from build123d import *

# Parameters (mm, degrees)
F0_W     = 127
F0_H     = 127
F1_DEPTH = 127
F2_W     = 38.1
F2_H     = 38.1
F3_DEPTH = 25.4
F4_W     = 88.9
F4_H     = 25.4
F5_DEPTH = 50.8
F6_W     = 25.4
F6_H     = 25.4
F7_DEPTH = 63.5
F8_W     = 12.7
F8_H     = 12.7
F9_DEPTH = 10.16


with BuildPart() as f1:
    # F0 (on Front) → F1 (new body)
    with BuildSketch(Plane.XZ):
        Rectangle(F0_W, F0_H)
    extrude(amount=F1_DEPTH)

    # F2 (on face) → F3 (join)
    with BuildSketch(Plane.XZ.offset(127)):
        with Locations((-44.45, -44.45)):
            Rectangle(F2_W, F2_H)
        with Locations((44.45, -44.45)):
            Rectangle(F2_W, F2_H)
    extrude(amount=F3_DEPTH)

    # F4 (on face) → F5 (join)
    with BuildSketch(Plane.XZ.offset(127)):
        with Locations((0, 76.2)):
            Rectangle(F4_W, F4_H)
        with Locations((0, 50.8)):
            Rectangle(F4_W, F4_H)
    extrude(amount=F5_DEPTH)

    # F6 (on face) → F7 (join)
    with BuildSketch(Plane.XY.offset(88.9)):
        with Locations((-31.75, -139.7)):
            Rectangle(F6_W, F6_H)
        with Locations((31.75, -139.7)):
            Rectangle(F6_W, F6_H)
    extrude(amount=F7_DEPTH)

    # F8 (on face) → F9 (join)
    with BuildSketch(Plane.XZ.offset(177.8)):
        with Locations((0, 62.430865)):
            Rectangle(F8_W, F8_H)
    extrude(amount=F9_DEPTH)


solid = f1.part
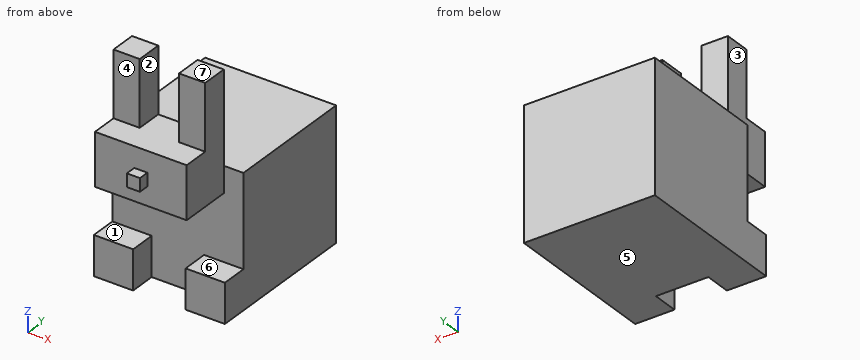
Read the model definition and answer for the solid it produces. Units are mm, in the model's axes. Face numbers are marked on the shaded views. A direction names the side the tool comes from. Coordinates: 2 decimals unless noted, no trailing zeros. Loops run counter-clockwise (first coordinate to the right, second up) from the corner with the lowest first, then second, coordinate; pieces in that order, holes last.
Q1. The part is cut by section B-B on z = 134. Write down the section's boundary in (x, y), and give its area (3 significant figures).
Q2. The mould has two halves that part along Z. Classify the marked faces 5, 6 and 7: +Z half, -Z half, draft (parallel to the pull), parting line (faces both ways), or undercut.
Q3. The part is cut by section D-D on y = -67. Write down the section's boundary in (x, z), and give its area (3 significant figures).
Q4. The part is cut by section A-A on y = -148.5. Write down the section's boundary in (x, z), and give its area (3 significant figures).
Q5. Which of the six approach directions +Z, -Z, +X, -X, +Y, -Y give full straight-line access (tool end or side, diameter ignored) to the marked faces 1, 2, 3 and 4?
Q6. Each of these flat-tipped pins is pushed along its axis until it touches: pin 1 Ø1 at (x, z) = (-2, -8) entering from -Y; pin 2 Ø3 at (y, z) = (-142, 50) entering from -X; pin 3 Ø11.5 at (x, z) = (-45, -38.5) entering from -Y. Where does it stop, or does it pass through?
Q7. Consider probe 1 along X at (y, z) = (-144, -37.5); probe 2 along Z at (x, y) = (-31.5, -157.5); probe 3 along Z at (x, y) = (-35, -146.5). Determine where each line is inside the solid, lowest interval first.
Q8. The part is cut by section C-C on x = -10. Write down the section's boundary in (y, z).
Results below:
1. outline: (-44.45, -152.4) - (-19.05, -152.4) - (-19.05, -127) - (-44.45, -127) - close; (19.05, -152.4) - (44.45, -152.4) - (44.45, -127) - (19.05, -127) - close
1. area: 1,290 mm2
2. face 5: -Z half
2. face 6: undercut
2. face 7: +Z half
3. outline: (-63.5, -63.5) - (63.5, -63.5) - (63.5, 63.5) - (-63.5, 63.5) - close
3. area: 16,100 mm2
4. outline: (-63.5, -63.5) - (-25.4, -63.5) - (-25.4, -25.4) - (-63.5, -25.4) - close; (-44.45, 38.1) - (44.45, 38.1) - (44.45, 152.4) - (19.05, 152.4) - (19.05, 88.9) - (-19.05, 88.9) - (-19.05, 152.4) - (-44.45, 152.4) - close; (25.4, -63.5) - (63.5, -63.5) - (63.5, -25.4) - (25.4, -25.4) - close
4. area: 10,600 mm2
5. face 1: +X, -X, -Y
5. face 2: +Z, +Y, -Y
5. face 3: +Z, -X, -Y
5. face 4: +Z, +X, -X, -Y
6. pin 1: stops at y = -127
6. pin 2: stops at x = -44.45
6. pin 3: stops at y = -152.4
7. probe 1: x = -63.5 to -25.4, 25.4 to 63.5
7. probe 2: z = 38.1 to 88.9
7. probe 3: z = -63.5 to -25.4, 38.1 to 152.4
8. outline: (-177.8, 38.1) - (-127, 38.1) - (-127, -63.5) - (0, -63.5) - (0, 63.5) - (-127, 63.5) - (-127, 88.9) - (-177.8, 88.9) - close
